For this review, take the finished solid that the model builds, in its own axes (mm). Face numbers are marked on the shaded views. Give positions to 0.01 mm unless a question says otherwise; leave off trailing zeros. Loops run counter-clockwise (first coordinate to the right, second up) from the corner with the lowest first, then second, coordinate; pieces in that order, holes last. Notation, with made-up numbers: (5.25, 7.25) - (43.25, 7.25) arc R23 cw to (43.25, 34.25) - close; hole circle Ø6 at (-39.75, 86). An arc over 180 degrees is marked (long way). Put each result on its own line as item: value.
from build123d import *

# Parameters (mm, degrees)
F0_W = 0.508
F0_H = 1.27


with BuildPart() as f1:
    # F0 (on Front) → F1 (revolve)
    with BuildSketch(Plane.XZ):
        Polygon((21.417418, 4.309946), (-35.478582, 4.309946), (-35.478582, 2.277946), (-25.318582, 2.277946), (-24.810582, 2.277946), (-18.206582, 2.277946), (-17.698582, 2.277946), (-11.094582, 2.277946), (-10.586582, 2.277946), (21.417418, 2.277946), align=None)
        with Locations((-25.064582, 1.642946)):
            Rectangle(F0_W, F0_H)
        with Locations((-10.840582, 1.642946)):
            Rectangle(F0_W, F0_H)
        with Locations((-17.952582, 1.642946)):
            Rectangle(F0_W, F0_H)
    revolve(axis=Axis((21.417418, 0, 3.293946), (0, 0, -1)))


solid = f1.part
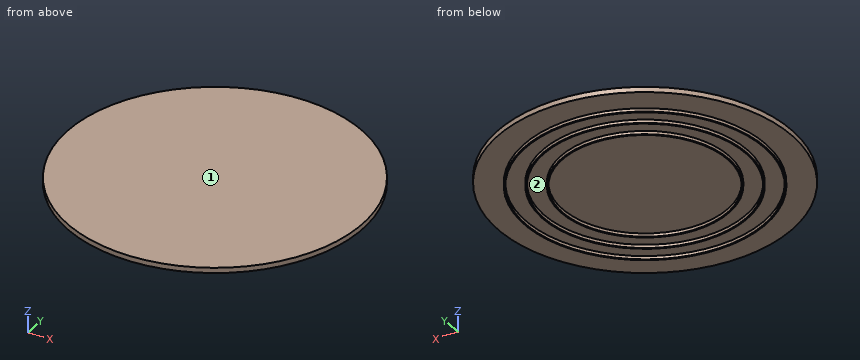
1) Take a section at D-D on y = -42.5. State the section outline as (x, z) points, and give its area (3 significant figures).
Geometry check:
outline: (-16.41, 2.28) - (1.98, 2.28) - (1.98, 1.01) - (3.23, 1.01) - (3.23, 2.28) - (39.6, 2.28) - (39.6, 1.01) - (40.86, 1.01) - (40.86, 2.28) - (59.24, 2.28) - (59.24, 4.31) - (-16.41, 4.31) - close
area: 157 mm²
2) Draft analysis for pull direction Y (two halves, no side actions). For the marked faces 1 and 2, state which applies: pulls with the +Y half, pulls with the -Y half, needs draft (parallel to the pull), parting line crosses it, or undercut.
Geometry check:
face 1: needs draft
face 2: undercut
3) Take a section at C-C on x = -3. State the section outline as (y, z) points, and give its area (3 significant figures).
Geometry check:
outline: (-51.39, 2.28) - (-39.85, 2.28) - (-39.85, 1.01) - (-39.25, 1.01) - (-39.25, 2.28) - (-31.21, 2.28) - (-31.21, 1.01) - (-30.56, 1.01) - (-30.56, 2.28) - (-21.47, 2.28) - (-21.47, 1.01) - (-20.69, 1.01) - (-20.69, 2.28) - (20.69, 2.28) - (20.69, 1.01) - (21.47, 1.01) - (21.47, 2.28) - (30.56, 2.28) - (30.56, 1.01) - (31.21, 1.01) - (31.21, 2.28) - (39.25, 2.28) - (39.25, 1.01) - (39.85, 1.01) - (39.85, 2.28) - (51.39, 2.28) - (51.39, 4.31) - (-51.39, 4.31) - close
area: 214 mm²
4) Take a section at B-B on y = 0. State the section outline as (x, z) points, and give its area (3 significant figures).
Geometry check:
outline: (-35.48, 2.28) - (-25.32, 2.28) - (-25.32, 1.01) - (-24.81, 1.01) - (-24.81, 2.28) - (-18.21, 2.28) - (-18.21, 1.01) - (-17.7, 1.01) - (-17.7, 2.28) - (-11.09, 2.28) - (-11.09, 1.01) - (-10.59, 1.01) - (-10.59, 2.28) - (53.42, 2.28) - (53.42, 1.01) - (53.93, 1.01) - (53.93, 2.28) - (60.53, 2.28) - (60.53, 1.01) - (61.04, 1.01) - (61.04, 2.28) - (67.65, 2.28) - (67.65, 1.01) - (68.15, 1.01) - (68.15, 2.28) - (78.31, 2.28) - (78.31, 4.31) - (-35.48, 4.31) - close
area: 235 mm²
5) Take a section at A-A on z = 1.65. State the section outline as (x, y) points, and give its area (3 significant figures).
Geometry check:
outline: circle Ø93.47 at (21.42, 0); circle Ø79.25 at (21.42, 0); circle Ø65.02 at (21.42, 0); hole circle Ø92.46 at (21.42, 0); hole circle Ø78.23 at (21.42, 0); hole circle Ø64.01 at (21.42, 0)
area: 377 mm²
6) Insertion check: pin 1 Ø1.5 at (x, z) = (1.5, 4) entering from +Y; pin 2 Ø1 at (y, z) = (-16, 3.5) entering from -X. Each pin has a flat end and moves straight along its axis. Give the tip position at first contact, or say it passes through.
Geometry check:
pin 1: stops at y = 53.57
pin 2: stops at x = -33.33
7) Wall thickness on line 1 (X direction, y = -17, z = 2.15); line 2 (Y direction, x = 39, z = 1.95); line 3 (Y direction, x = 1, z = 1.6): over which ranges is each line inside the solid? List them lowest first.
Geometry check:
line 1: x = -22.12 to -21.57, -14.37 to -13.81, -6.3 to -5.7, 48.53 to 49.13, 56.65 to 57.21, 64.41 to 64.95
line 2: y = -43.3 to -42.75, -35.51 to -34.94, -27.35 to -26.74, 26.74 to 27.35, 34.94 to 35.51, 42.75 to 43.3
line 3: y = -42.04 to -41.47, -33.96 to -33.36, -25.3 to -24.65, 24.65 to 25.3, 33.36 to 33.96, 41.47 to 42.04
